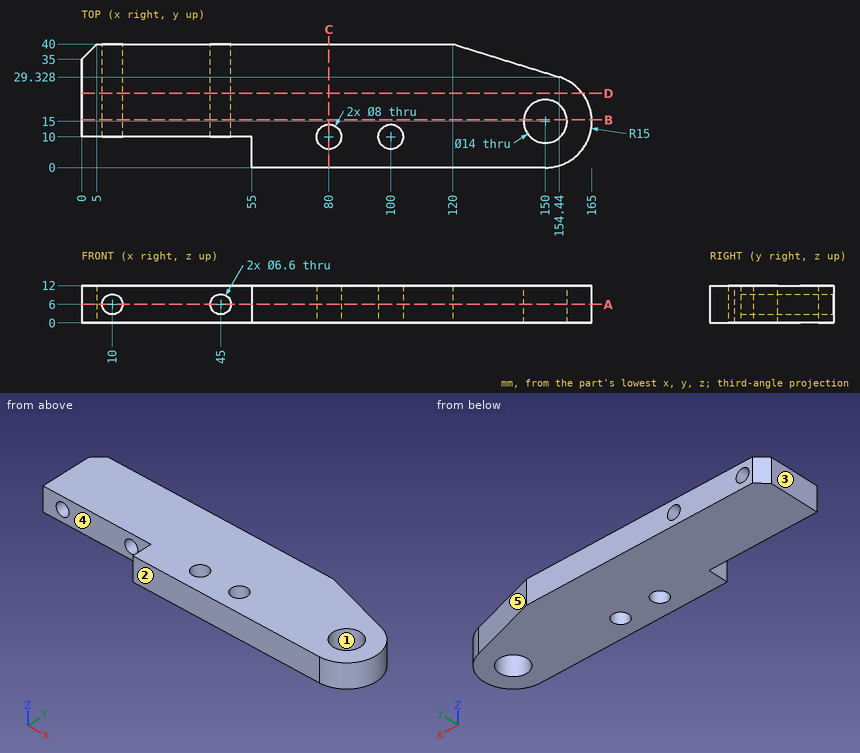
Source: three-view drawing plus pictorial views. Frame: mm from the lowest corner of the part. A direction names the side the tool comes from. Coordinates: 2 decimals unless noted, no trailing zeros. Order: outer loops, then holes, each group sorted by start corner. A loop starts at its lowest first (then second) coordinate and runs counter-clockwise, first axis right, second up. Notation, with made-up numbers: (39.5, -1) -> (85.5, -1) arc R20 ccw to (85.5, 12) -> close; hole circle Ø3 at (61, 29). An arc over 180 degrees is marked (long way). Write item = value, one per line.
(1) Pin query (flat end, axial travel): pin 1 Ø12.5 at (x, y) = (150, 15) entering from +Z; pin 2 Ø13 at (x, y) = (100, 10) entering from +Z; pin 3 Ø3 at (y, z) = (22, 8) entering from +X; pin 4 Ø1.5 at (y, z) = (7.5, 7.5) entering from -X. Return the tip coordinate at first contact, or that it passes through.
Solved:
pin_1 = through
pin_2 = 12
pin_3 = 163.96
pin_4 = 55
(2) Pull-direction query (Y, two-part tool) for the marked faces 1, 2 and 3; classes: pulls with the +Y half, pulls with the -Y half, needs draft (parallel to the pull), parting line crosses it, or undercut.
Solved:
face_1 = undercut
face_2 = pulls with the -Y half
face_3 = needs draft
(3) Cut plane B-B on y = 15.5. Return loops of the section in (x, z).
Solved:
outline = (0, 0) -> (143.02, 0) -> (143.02, 12) -> (0, 12) -> close; (156.98, 0) -> (164.99, 0) -> (164.99, 12) -> (156.98, 12) -> close; hole circle Ø6.6 at (10, 6); hole circle Ø6.6 at (45, 6)
(4) Cut plane A-A on z = 6. Return loops of the section in (x, y).
Solved:
outline = (0, 10) -> (6.7, 10) -> (6.7, 40) -> (5, 40) -> (0, 35) -> close; (13.3, 10) -> (41.7, 10) -> (41.7, 40) -> (13.3, 40) -> close; (48.3, 10) -> (55, 10) -> (55, 0) -> (150, 0) arc R15 ccw to (154.44, 29.33) -> (120, 40) -> (48.3, 40) -> close; hole circle Ø8 at (80, 10); hole circle Ø8 at (100, 10); hole circle Ø14 at (150, 15)
(5) Access query for the marked faces 4 and 5. Directions: +Z, -Z, +X, -X, +Y, -Y. A direction counts if a zero-diameter tool reaches every point of the face in a straight line with its end or side. Return the directions, or none.
Solved:
face_4 = +Z, -Z, -X, -Y
face_5 = +Z, -Z, +X, +Y
(6) Line query: line 1 (Z direction, x = 45, y = 16); line 2 (X direction, y = 15.5, z = 8.75); line 3 (X direction, y = 15, z = 5) (1 decimal). Output: solid intervals per line, ascending.
Solved:
line_1 = 0 to 2.7, 9.3 to 12
line_2 = 0 to 8.18, 11.82 to 43.18, 46.82 to 143.02, 156.98 to 164.99
line_3 = 0 to 6.9, 13.1 to 41.9, 48.1 to 143, 157 to 165
(7) Cut plane D-D on y = 24. Return loops of the section in (x, z), plus the area to 3 significant figures.
Solved:
outline = (0, 0) -> (162, 0) -> (162, 12) -> (0, 12) -> close; hole circle Ø6.6 at (10, 6); hole circle Ø6.6 at (45, 6)
area = 1,880 mm²
(8) Cut plane C-C on x = 80. Return loops of the section in (y, z).
Solved:
outline = (0, 0) -> (6, 0) -> (6, 12) -> (0, 12) -> close; (14, 0) -> (40, 0) -> (40, 12) -> (14, 12) -> close
